For this review, take the finished solid that the model builds, in its own axes (mm). A direction names the side the tool comes from. Give positions to 0.01 mm unless a question says otherwise; leave off trailing zeros. Loops run counter-clockwise (first coordinate to the right, second up) from the corner with the lowest first, then second, coordinate; pieces in that order, holes last. Notation, with made-up numbers: (-1, 75) - (16, 75) arc R28 cw to (16, 94) - close; hole circle Ø1 at (14.25, -0.75). An arc over 180 degrees is marked (long way). Answer in a Markdown table with one row per item.
```python
from build123d import *

# Parameters (mm, degrees)
BOSS_EXTRUDE1_DEPTH        = 5
F_3_2_3_2_DIAMETER_HOLE1_D = 3.2
BOSS_EXTRUDE2_DEPTH        = 5
SKETCH10_W                 = 7
SKETCH10_H                 = 7
CUT_EXTRUDE2_DEPTH         = 2.6
SKETCH11_R                 = 2.1
CUT_EXTRUDE3_DEPTH         = 41.33014714


with BuildPart() as part:
    # Sketch1 → Boss-Extrude1 (new body)
    with BuildSketch(Plane(origin=(0, 0, 0), x_dir=(1, 0, 0), z_dir=(0, 1, 0))):
        with BuildLine():
            Line((-216.657705663, 38.202599087), (-206.809628133, 36.46611731))
            ThreePointArc((-206.809628133, 36.46611731), (-210, 0), (-206.809628133, -36.46611731))
            Line((-206.809628133, -36.46611731), (-216.657705663, -38.202599087))
            ThreePointArc((-216.657705663, -38.202599087), (-220, 0), (-216.657705663, 38.202599087))
        make_face()
    extrude(amount=BOSS_EXTRUDE1_DEPTH)

    # Ø3.2 (3.2) Diameter Hole1 (through all)
    with Locations(Plane(origin=(0, 0, 0), x_dir=(-1, 0, 0), z_dir=(0, -1, 0))):
        with Locations((214.18186009, -18.738484691), (214.18186009, 18.738484691), (213.160645195, -28.063131327), (213.160645195, 28.063131327)):
            Hole(F_3_2_3_2_DIAMETER_HOLE1_D / 2)

    # Sketch9 → Boss-Extrude2 (add)
    with BuildSketch(Plane(origin=(0, 5, 0), x_dir=(1, 0, 0), z_dir=(0, 1, 0))):
        with BuildLine():
            Line((-219.772609758, 10), (-209.761769634, 10))
            ThreePointArc((-209.761769634, 10), (-210, 0), (-209.761769634, -10))
            Line((-209.761769634, -10), (-219.772609758, -10))
            ThreePointArc((-219.772609758, -10), (-220, 0), (-219.772609758, 10))
        make_face()
    extrude(amount=BOSS_EXTRUDE2_DEPTH)

    # Sketch10 → Cut-Extrude2 (cut)
    with BuildSketch(Plane.ZY.offset(215)):
        with Locations((0, 10)):
            Rectangle(SKETCH10_W, SKETCH10_H)
    extrude(amount=CUT_EXTRUDE2_DEPTH, mode=Mode.SUBTRACT)

    # Sketch11 → Cut-Extrude3 (cut, through all)
    with BuildSketch(Plane.ZY.offset(215)):
        with Locations((0, 10)):
            Circle(SKETCH11_R)
    extrude(amount=CUT_EXTRUDE3_DEPTH, mode=Mode.SUBTRACT)


solid = part.part
```
1. Clearance check with flat-ended pins moving along their axes: pin 1 (3 mm diameter, centred on x = -217, y = 8, fed in from +Z); pin 2 (1.8 mm diameter, centred on y = 7.5, z = -1.5, fed in from +X); pin 3 (2.5 mm diameter, centred on x = -213.16, z = 28.06, fed in from -Y) (1 decimal); pin 4 (3.5 mm diameter, centred on x = -214.18, z = -18.74, fed in from +Y). State where each tip first meets the part, or that it passes through.
Values:
| item | result |
|---|---|
| pin 1 | stops at z = 10 |
| pin 2 | stops at x = -209.99 |
| pin 3 | passes through |
| pin 4 | stops at y = 5 |
2. Wall thickness on line 1 (Z direction, x = -217.5, y = 9.5); line 2 (Z direction, x = -213.5, y = 8.25); line 3 (Y direction, x = -216.5, z = 32): over which ranges is each line inside the solid? List them lowest first. Write a range as [from, to].
Values:
| item | result |
|---|---|
| line 1 | z = [-10, -3.5], [3.5, 10] |
| line 2 | z = [-10, 10] |
| line 3 | y = [0, 5] |
3. For faces 4 (the face through (-213, 5, -24)), 5 (the face through (-213, 5, 24)), 6 (the face through (-218.8, 7.9, 0)), 7 (the face through (-217.6, 7, 0)), 8 (the face through (-211.635, 2.535, 27.583)), list the 3-axis set-ups (+Z, -Z, +X, -X, +Y, -Y) from which the entire face can be reached by the end or side of a thin tool; tool diameter is ignored.
Values:
| item | result |
|---|---|
| face 4 | -Z, +X, -X, +Y |
| face 5 | +Z, +X, -X, +Y |
| face 6 | -X, +Y |
| face 7 | +Y |
| face 8 | +Y, -Y |
4. We need section C-C, the plane x = -209. Give the boundary of the cut face in (y, z), and give its area (3 significant figures).
Values:
| item | result |
|---|---|
| outline | (0, -36.85) - (5, -36.85) - (5, -20.47) - (0, -20.47) - close; (0, 20.47) - (5, 20.47) - (5, 36.85) - (0, 36.85) - close |
| area | 164 mm^2 |
5. We need section B-B, the plane z = 0. Give the boundary of the cut face in (x, y), and give its area (3 significant figures).
Values:
| item | result |
|---|---|
| outline | (-220, 0) - (-210, 0) - (-210, 10) - (-215, 10) - (-215, 6.5) - (-217.6, 6.5) - (-217.6, 7.9) - (-220, 7.9) - close |
| area | 85.9 mm^2 |
6. We need section A-A, the plane y = 1.75. Give the boundary of the cut face in (x, z).
Values:
| item | result |
|---|---|
| outline | (-216.66, -38.2) - (-206.81, -36.47) arc R210 cw to (-206.81, 36.47) - (-216.66, 38.2) arc R220 ccw to start; hole circle Ø3.2 at (-214.18, -18.74); hole circle Ø3.2 at (-214.18, 18.74); hole circle Ø3.2 at (-213.16, -28.06); hole circle Ø3.2 at (-213.16, 28.06) |
7. Mouldability with a two-part tool opening along Z and no side actions: class faces 1 (the face through (-215, 7, 10)), 2 (the face through (-216, 8, -3.5)), 3 (the face through (-215, 7, -10)) as released by +Z, released by -Z, zero draft, split by the parting line, or undercut.
Values:
| item | result |
|---|---|
| face 1 | released by +Z |
| face 2 | undercut |
| face 3 | released by -Z |
8. We need section D-D, the plane y = 9. Give the boundary of the cut face in (x, z), and give its area (3 significant figures).
Values:
| item | result |
|---|---|
| outline | (-219.99, -1.85) arc R220 ccw to (-219.77, -10) - (-209.76, -10) arc R210 cw to (-209.76, 10) - (-219.77, 10) arc R220 ccw to (-219.99, 1.85) - (-217.6, 1.85) - (-217.6, 3.5) - (-215, 3.5) - (-215, -3.5) - (-217.6, -3.5) - (-217.6, -1.85) - close |
| area | 173 mm^2 |
